Geometry check sheet. Reference: the model listing, model coordinates, mm. Round coordinates to 2 decimals unless told otherwise and drop trailing zeros. Write each loop counter-clockwise with the first axis right and the second up, starting at its lowest first coordinate (ties: lowest second). Pieces come first, ordered by that corner, then holes. Notation, with made-up numbers: (54.25, 81) -> (107.25, 81) arc R22 cw to (107.25, 102) -> close; hole circle Ø5 at (57, -16.75). An arc over 180 degrees is marked (long way). Use a Markdown table: item, result.
```python
from build123d import *

# Parameters (mm, degrees)
SKETCH1_W                  = 19.05
SKETCH1_H                  = 11.43
BOSS_EXTRUDE1_DEPTH        = 12.7
SKETCH3_R                  = 3.175
CUT_EXTRUDE1_DEPTH         = 17.872369425
F_10_32_TAPPED_HOLE3_D     = 4.0386
F_10_32_TAPPED_HOLE3_DEPTH = 7.45744
F_10_32_TAPPED_HOLE3_TIP   = 1.213317848


with BuildPart() as part:
    # Sketch1 → Boss-Extrude1 (new body)
    with BuildSketch(Plane.XY):
        Rectangle(SKETCH1_W, SKETCH1_H)
    extrude(amount=BOSS_EXTRUDE1_DEPTH)

    # Sketch3 → Cut-Extrude1 (cut, through all)
    with BuildSketch(Plane.XY.offset(12.7)):
        with Locations((3.175, 0)):
            Circle(SKETCH3_R)
    extrude(amount=-CUT_EXTRUDE1_DEPTH, mode=Mode.SUBTRACT)

    # #10-32 Tapped Hole3
    with Locations(Plane(origin=(-9.525, 0, 6.35), x_dir=(0, 0, -1), z_dir=(-1, 0, 0))):
        with Locations((0, 0)):
            Hole(F_10_32_TAPPED_HOLE3_D / 2, depth=F_10_32_TAPPED_HOLE3_DEPTH)
            with Locations((0, 0, -(F_10_32_TAPPED_HOLE3_DEPTH + F_10_32_TAPPED_HOLE3_TIP / 2))):  # 118° drill point
                Cone(0, F_10_32_TAPPED_HOLE3_D / 2, F_10_32_TAPPED_HOLE3_TIP, mode=Mode.SUBTRACT)


solid = part.part
```
(1) Section check A-A on x = -8. Record the cut outline in (y, z) (3 decimals), plus the area to 3 significant figures.
A:
| item | result |
|---|---|
| outline | (-5.715, 0) -> (5.715, 0) -> (5.715, 12.7) -> (-5.715, 12.7) -> close; hole circle Ø4.039 at (0, 6.35) |
| area | 132 mm2 |
(2) Section check B-B on y = -2.5. Record the cut outline in (x, z) (3 decimals).
A:
| item | result |
|---|---|
| outline | (-9.525, 0) -> (1.218, 0) -> (1.218, 12.7) -> (-9.525, 12.7) -> close; (5.132, 0) -> (9.525, 0) -> (9.525, 12.7) -> (5.132, 12.7) -> close |
(3) Release check for a two-part mould opening along Z. For faces 1 (the face through (-5.744, -0.607, 8.276)), 2 (the face through (0, 1, 12.7)), 3 (the face through (0, 1, 0)) record: +Z half, -Z half, draft (parallel to the pull), parting line (faces both ways), or undercut.
A:
| item | result |
|---|---|
| face 1 | undercut |
| face 2 | +Z half |
| face 3 | -Z half |
(4) Thickness scan on line 1 (Y direction, x = -5.5, z = 6.35) (3 decimals); line 2 (Y direction, x = -3.5, z = 5) (3 decimals); line 3 (X direction, y = -1.5, z = 10.5) (3 decimals). Record the ranges inside material, lowest first.
A:
| item | result |
|---|---|
| line 1 | y = -5.715 to -2.019, 2.019 to 5.715 |
| line 2 | y = -5.715 to -1.502, 1.502 to 5.715 |
| line 3 | x = -9.525 to 0.377, 5.973 to 9.525 |
(5) Section check C-C on x = 4.5. Record the cut outline in (y, z) (3 decimals), plus the area to 3 significant figures.
A:
| item | result |
|---|---|
| outline | (-5.715, 0) -> (-2.885, 0) -> (-2.885, 12.7) -> (-5.715, 12.7) -> close; (2.885, 0) -> (5.715, 0) -> (5.715, 12.7) -> (2.885, 12.7) -> close |
| area | 71.9 mm2 |
(6) Gauge pin test, flat end, axial feed: pin 1 Ø5.5 at (x, y) = (3.175, 0) entering from -Z. Record the tip position at first contact, or that the pin passes through.
A:
| item | result |
|---|---|
| pin 1 | passes through |
